```python
from build123d import *

# Parameters (mm, degrees)
F0_W     = 10
F0_H     = 10
F1_DEPTH = 144
F2_W     = 10
F2_H     = 5
F3_DEPTH = 10
F4_SIZE  = 9.99999


# Not quite as in the source:
# - a fillet or chamfer is up to 0.001 mm smaller than in the source, because OpenCascade refuses the exact size


with BuildPart() as f1:
    # F0 (on Front) → F1 (new body)
    with BuildSketch(Plane.XZ):
        Rectangle(F0_W, F0_H)
    extrude(amount=F1_DEPTH)

    # F2 (on face) → F3 (cut)
    with BuildSketch(Plane.YZ.offset(5)):
        with Locations((-5, 2.5)):
            Rectangle(F2_W, F2_H)
    extrude(amount=-F3_DEPTH, mode=Mode.SUBTRACT)

    # F4 (size 10 in the source; OpenCascade refuses exactly that, so slightly less here)
    f4_edges = [f1.edges().sort_by_distance(p)[0] for p in [
        (5, -144, 0),
    ]]
    chamfer(f4_edges, length=F4_SIZE)


solid = f1.part
```
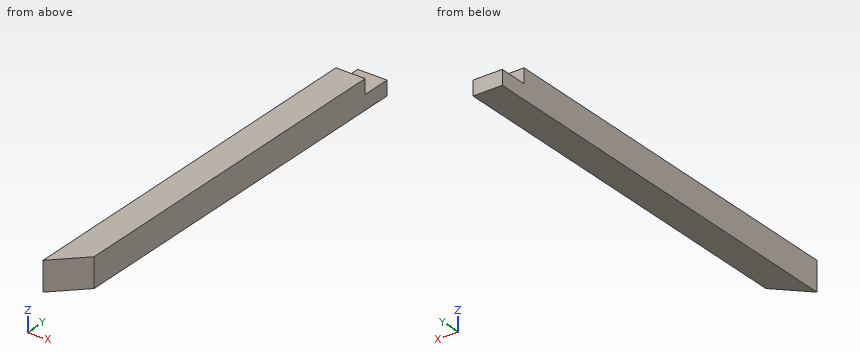
Design review of the part built by this model. Coordinates are the model's own, in mm. Coordinates: 2 decimals unless noted, no trailing zeros. Order: outer loops, then holes, each group sorted by start corner. A loop starts at its lowest first (then second) coordinate and runs counter-clockwise, first axis right, second up.
1) Take a section at B-B, the plane x = 2.5. Give the boundary of the cut face in (y, z), and give its area (4 significant figures).
2) Clearance check with a flat-ended pin moving along its axis: pin 1 (1 mm diameter, centred on x = -0.5, z = 3, fed in from -Y). State where the tip first meets the part, or that it passes through.
3) Wall thickness on line 1 along Y through (x, z) = (-3.5, 4.5); line 2 along Y through (x, z) = (-4, -1.5): over which ranges is each line inside the solid? List them lowest first.
Returned:
1. outline: (-136.5, -5) - (0, -5) - (0, 0) - (-10, 0) - (-10, 5) - (-136.5, 5) - close
1. area: 1,315 mm2
2. pin 1: stops at y = -140
3. line 1: y = -142.5 to -10
3. line 2: y = -143 to 0
